from build123d import *

# Parameters (mm, degrees)
ESQUISSE1_W             = 60
ESQUISSE1_H             = 50
BOSS_EXTRU_2_DEPTH      = 14.1
ESQUISSE2_R             = 1.5
ESQUISSE2_W             = 2.5
ESQUISSE2_H             = 2.5
ENL_V_MAT_EXTRU_1_DEPTH = 42.518790927


with BuildPart() as part:
    # Esquisse1 → Boss.-Extru.2 (new body)
    with BuildSketch(Plane(origin=(0, 0, 0), x_dir=(1, 0, 0), z_dir=(0, 1, 0))):
        Rectangle(ESQUISSE1_W, ESQUISSE1_H)
    extrude(amount=BOSS_EXTRU_2_DEPTH)

    # Esquisse2 → Enlèv. mat.-Extru.1 (cut, through all)
    with BuildSketch(Plane(origin=(0, 14.1, 0), x_dir=(1, 0, 0), z_dir=(0, 1, 0))):
        with Locations(Location((-9.25, 10.25, 0), (0, 0, 270))):
            Circle(ESQUISSE2_R)
        with Locations(Location((9.25, 10.25, 0), (0, 0, 270))):
            Circle(ESQUISSE2_R)
        with Locations(Location((9.25, -10.25, 0), (0, 0, 90))):
            Circle(ESQUISSE2_R)
        with Locations(Location((-9.25, -10.25, 0), (0, 0, 90))):
            Circle(ESQUISSE2_R)
        with Locations((3.81, -10.25)):
            Rectangle(ESQUISSE2_W, ESQUISSE2_H)
        with Locations((-3.81, 10.25)):
            Rectangle(ESQUISSE2_W, ESQUISSE2_H)
        with Locations((1.27, -10.25)):
            Rectangle(ESQUISSE2_W, ESQUISSE2_H)
        with Locations((-1.27, 10.25)):
            Rectangle(ESQUISSE2_W, ESQUISSE2_H)
        with Locations((1.27, 10.25)):
            Rectangle(ESQUISSE2_W, ESQUISSE2_H)
        with Locations((3.81, 10.25)):
            Rectangle(ESQUISSE2_W, ESQUISSE2_H)
        with Locations((-1.27, -10.25)):
            Rectangle(ESQUISSE2_W, ESQUISSE2_H)
        with Locations((-3.81, -10.25)):
            Rectangle(ESQUISSE2_W, ESQUISSE2_H)
    extrude(amount=-ENL_V_MAT_EXTRU_1_DEPTH, mode=Mode.SUBTRACT)


solid = part.part
Can you work these out from the model? Positions are in its coordinate system, mm. Give positions to 0.01 mm unless a question says otherwise; leave off trailing zeros. Loops run counter-clockwise (first coordinate to the right, second up) from the corner with the lowest first, then second, coordinate; pieces in that order, holes last. Notation, with made-up numbers: (-39.75, 78) -> (3.25, 78) arc R18 ccw to (3.25, 95) -> close; hole circle Ø2 at (16.25, 48.25). An arc over 180 degrees is marked (long way). Write item = value, one per line.
1) I need wall thicknesses on L1, parallel to Z at x = -4, y = 0.75. Which ranges of the line are inside material? Lowest first, please. Write a range as from..to.
Check result:
L1 = -25..-11.5, -9..9, 11.5..25
2) Thinking about a two-plate mould opening in X: for faces 1 (the flat face through (-4, 7, -9)), 2 (the flat face through (0, 0, 0)), 3 (the flat face through (30, 7, 0)), which applies, released by +X, released by -X, zero draft, split by the parting line, or undercut?
Check result:
face_1 = undercut
face_2 = zero draft
face_3 = released by +X
3) Suppose I cut it at B-B on x = 9.25. Write out the boundary of the cut face in (y, z).
Check result:
outline = (0, -25) -> (14.1, -25) -> (14.1, -11.75) -> (0, -11.75) -> close; (0, -8.75) -> (14.1, -8.75) -> (14.1, 8.75) -> (0, 8.75) -> close; (0, 11.75) -> (14.1, 11.75) -> (14.1, 25) -> (0, 25) -> close
4) Suppose I cut it at A-A on z = -10.25. Write out the boundary of the cut face in (x, y), then the cut area to 3 significant figures.
Check result:
outline = (-30, 0) -> (-10.75, 0) -> (-10.75, 14.1) -> (-30, 14.1) -> close; (-7.75, 0) -> (-5.06, 0) -> (-5.06, 14.1) -> (-7.75, 14.1) -> close; (-2.56, 0) -> (-2.52, 0) -> (-2.52, 14.1) -> (-2.56, 14.1) -> close; (-0.02, 0) -> (0.02, 0) -> (0.02, 14.1) -> (-0.02, 14.1) -> close; (2.52, 0) -> (2.56, 0) -> (2.56, 14.1) -> (2.52, 14.1) -> close; (5.06, 0) -> (7.75, 0) -> (7.75, 14.1) -> (5.06, 14.1) -> close; (10.75, 0) -> (30, 0) -> (30, 14.1) -> (10.75, 14.1) -> close
area = 620 mm2
5) Suppose I cut it at C-C on y = 12.5. Give the number of separate pieces and of enclosed holes in the cut face, then the cut area to 3 significant figures.
Check result:
separate_pieces = 1
enclosed_holes = 12
area = 2,920 mm2
